from build123d import *

# Parameters (mm, degrees)
SKETCH_1_R          = 3.5
SKETCH_1_R_2        = 1.5
EXTRUDE_1_DEPTH     = 4
SKETCH_2_R          = 3
CUT_EXTRUDE_1_DEPTH = 2
CUT_EXTRUDE_START   = -1
SKETCH_3_R          = 3
CUT_EXTRUDE_2_DEPTH = 1
EXTRUDE_START       = -1
SKETCH_4_R          = 2
EXTRUDE_2_DEPTH     = 1


with BuildPart() as part:
    # 草图1 → 凸台-拉伸1 (new body)
    with BuildSketch(Plane(origin=(0, 0, 0), x_dir=(1, 0, 0), z_dir=(0, 1, 0))):
        with Locations(Location((0, 0, 0), (0, 0, 270))):
            Circle(SKETCH_1_R)
        with Locations(Location((0, 0, 0), (0, 0, 270))):
            Circle(SKETCH_1_R_2, mode=Mode.SUBTRACT)
    extrude(amount=EXTRUDE_1_DEPTH)

    # 草图2 → 切除-拉伸1 (cut)
    with BuildSketch(Plane.XZ):
        with Locations(Location((0, 0, 0), (0, 0, 270))):
            Circle(SKETCH_2_R)
    extrude(amount=-CUT_EXTRUDE_1_DEPTH, mode=Mode.SUBTRACT)

    # 草图3 → 切除-拉伸2 (cut)
    with BuildSketch(Plane(origin=(0, 4, 0), x_dir=(1, 0, 0), z_dir=(0, 1, 0)).offset(CUT_EXTRUDE_START)):
        with Locations(Location((0, 0, 0), (0, 0, 90))):
            Circle(SKETCH_3_R)
    extrude(amount=CUT_EXTRUDE_2_DEPTH, mode=Mode.SUBTRACT)

    # 草图4 → 凸台-拉伸2 (add)
    with BuildSketch(Plane(origin=(0, 4, 0), x_dir=(1, 0, 0), z_dir=(0, 1, 0)).offset(EXTRUDE_START)):
        with BuildLine():
            ThreePointArc((-2.449489743, -2.5), (-3.5, 0), (-2.449489743, 2.5))
            Line((-2.449489743, 2.5), (-14.086174253, 1.998142637))
            ThreePointArc((-14.086174253, 1.998142637), (-12.61658909, 1.444359461), (-12, 0))
            ThreePointArc((-12, 0), (-12.61658909, -1.444359461), (-14.086174253, -1.998142637))
            Line((-14.086174253, -1.998142637), (-2.449489743, -2.5))
        make_face()
        with BuildLine():
            ThreePointArc((14.086174253, -1.998142637), (12, 0), (14.086174253, 1.998142637))
            Line((14.086174253, 1.998142637), (2.449489743, 2.5))
            ThreePointArc((2.449489743, 2.5), (3.226702194, 1.355873501), (3.5, 0))
            ThreePointArc((3.5, 0), (3.226702194, -1.355873501), (2.449489743, -2.5))
            Line((2.449489743, -2.5), (14.086174253, -1.998142637))
        make_face()
        with Locations((-14, 0)):
            Circle(SKETCH_4_R)
        with Locations((14, 0)):
            Circle(SKETCH_4_R)
    extrude(amount=EXTRUDE_2_DEPTH)


solid = part.part
Design review of the part built by this model. Coordinates are the model's own, in mm. A direction names the side the tool comes from. Round coordinates to 2 decimals unless told otherwise and drop trailing zeros. Write each loop counter-clockwise with the first axis right and the second up, starting at its lowest first coordinate (ties: lowest second). Pieces come first, ordered by that corner, then holes.
Item 1: Consider section D-D on x = 5. Give the boundary of the cut face in (y, z), and give its area (3 significant figures).
Item 2: Consider section B-B on z = 0. Give the boundary of the cut face in (x, y), and give its area (3 significant figures).
Item 3: Consider section A-A on x = 0. Give the boundary of the cut face in (y, z), and give its area (3 significant figures).
Item 4: For pin 1 Ø1.5 at (x, z) = (-10.5, -3) entering from -Y; pin 2 Ø4 at (x, z) = (0, 0) entering from -Y; pin 3 Ø4 at (x, z) = (9, 0) entering from -Y; pin 4 Ø1 at (x, y) = (6.5, 3) entering from +Z, all flat-tipped, find the tip position at first contact; note any pin that passes through.
Item 5: Consider section C-C on y = 3.5. Give the boundary of the cut face in (x, z), and give its area (3 significant figures).
Item 6: Wall thickness on L1, parallel to X at y = 3.5, z = 0; L2, parallel to Z at x = 0, y = 2.5: over which ranges is each line inside the solid? List them lowest first.
Item 7: For faces 1 (the flat face through (1.3, 3, -1.3)), 2 (the cylindrical face through (0.154, 1.972, -3.497)), 3 (the flat face through (1, 0, 3)), list the 3-axis set-ups (+Z, -Z, +X, -X, +Y, -Y) from which the entire face can be reached by the end or side of a thin tool; tool diameter is ignored.
Item 8: Draft analysis for pull direction X (two halves, no side actions). For faces 4 (the flat face through (-1.3, 2, -1.3)), 5 (the flat face through (8.186, 3.493, 2.253)), 6 (the flat face through (-9, 3, 0)), 7 (the cylindrical face through (0.9, 0.99, -2.86)), state which applies: released by +X, released by -X, zero draft, split by the parting line, or undercut.
Check values:
1. outline: (3, -2.39) - (4, -2.39) - (4, 2.39) - (3, 2.39) - close
1. area: 4.78 mm2
2. outline: (-16, 3) - (-3.5, 3) - (-3.5, 0) - (-3, 0) - (-3, 2) - (-1.5, 2) - (-1.5, 3) - (-3, 3) - (-3, 4) - (-16, 4) - close; (1.5, 2) - (3, 2) - (3, 0) - (3.5, 0) - (3.5, 3) - (16, 3) - (16, 4) - (3, 4) - (3, 3) - (1.5, 3) - close
2. area: 32.0 mm2
3. outline: (0, -3.5) - (4, -3.5) - (4, -3) - (3, -3) - (3, -1.5) - (2, -1.5) - (2, -3) - (0, -3) - close; (0, 3) - (2, 3) - (2, 1.5) - (3, 1.5) - (3, 3) - (4, 3) - (4, 3.5) - (0, 3.5) - close
3. area: 7.00 mm2
4. pin 1: passes through
4. pin 2: stops at y = 2
4. pin 3: stops at y = 3
4. pin 4: stops at z = 2.35
5. outline: (-14.09, -2) - (-2.45, -2.5) arc R3.5 ccw to (2.45, -2.5) - (14.09, -2) arc R2 ccw to (14.09, 2) - (2.45, 2.5) arc R3.5 ccw to (-2.45, 2.5) - (-14.09, 2) arc R2 ccw to start; hole circle Ø6 at (0, 0)
5. area: 120 mm2
6. L1: x = -16 to -3, 3 to 16
6. L2: z = -3.5 to -1.5, 1.5 to 3.5
7. face 1: +Y
7. face 2: -Y
7. face 3: +Z, -Z, +X, -X, -Y
8. face 4: undercut
8. face 5: released by +X
8. face 6: zero draft
8. face 7: undercut
